The listing builds one solid part. Answer for the finished solid, in the listing's coordinates (mm). A direction names the side the tool comes from. Coordinates: 2 decimals unless noted, no trailing zeros. Order: outer loops, then holes, each group sorted by start corner. A loop starts at its lowest first (then second) coordinate and runs counter-clockwise, first axis right, second up. Notation, with made-up numbers: (-33, 58.5) -> (7, 58.5) arc R29 cw to (7, 89.5) -> close; hole circle Ø2 at (-3.75, -38). An arc over 180 degrees is marked (long way). Write item = value, one per line.
from build123d import *

# Parameters (mm, degrees)
CUT_EXTRUDE_1_DEPTH = 0.75


with BuildPart() as part:
    # 草图1 → 旋转1 (revolve)
    with BuildSketch(Plane.XY):
        Polygon((0, 0), (0, 1.25), (-9.75, 1.25), (-9.75, 0.875), (-10.5, 0.875), (-11.8, 2.35), (-12, 2.35), (-12, 0), align=None)
    revolve(axis=Axis((0, 0, 0), (-1, 0, 0)))

    # 草图2 → 切除-拉伸1 (cut)
    with BuildSketch(Plane.ZY.offset(12)):
        with BuildLine():
            Line((-0.3125, 1.5), (0.3125, 1.5))
            Line((0.3125, 1.5), (0.3125, 0.5625))
            ThreePointArc((0.3125, 0.5625), (0.385723305, 0.385723305), (0.5625, 0.3125))
            Line((0.5625, 0.3125), (1.5, 0.3125))
            Line((1.5, 0.3125), (1.5, -0.3125))
            Line((1.5, -0.3125), (0.5625, -0.3125))
            ThreePointArc((0.5625, -0.3125), (0.385723305, -0.385723305), (0.3125, -0.5625))
            Line((0.3125, -0.5625), (0.3125, -1.5))
            Line((0.3125, -1.5), (-0.3125, -1.5))
            Line((-0.3125, -1.5), (-0.3125, -0.5625))
            ThreePointArc((-0.3125, -0.5625), (-0.385723305, -0.385723305), (-0.5625, -0.3125))
            Line((-0.5625, -0.3125), (-1.5, -0.3125))
            Line((-1.5, -0.3125), (-1.5, 0.3125))
            Line((-1.5, 0.3125), (-0.5625, 0.3125))
            ThreePointArc((-0.5625, 0.3125), (-0.385723305, 0.385723305), (-0.3125, 0.5625))
            Line((-0.3125, 0.5625), (-0.3125, 1.5))
        make_face()
    extrude(amount=-CUT_EXTRUDE_1_DEPTH, mode=Mode.SUBTRACT)


solid = part.part
Q1. Each of these flat-tipped pins is pushed along its axis until it touches: pin 1 Ø2 at (x, y) = (-7, 0.5) entering from +Z; pin 2 Ø0.6 at (x, y) = (-11.5, 1) entering from -Z; pin 3 Ø0.5 at (x, y) = (-11.5, 0) entering from -Z. Where does it stop, or does it pass through?
The answers:
pin_1 = 1.25
pin_2 = -2.15
pin_3 = -2.29
Q2. Section C-C, the plane x = -6 is taken. Give the vertices of the cut face in (y, z).
The answers:
outline = circle Ø2.5 at (0, 0)
Q3. Find the intervals of material crossed by line 1 along Y through (x, z) = (-11.5, 1.25); line 2 along X through (y, z) = (-0.2, -1.05); line 3 along Y through (x, z) = (-8.75, 0), in increasing order.
The answers:
line_1 = -1.57 to -0.31, 0.31 to 1.57
line_2 = -11.25 to -10.67, -9.75 to 0
line_3 = -1.25 to 1.25
Q4. The mould has two halves that part along Z. Classify faces 3 (the face through (0, 0, 0)), 4 (the face through (-11.25, 0, 0)), 5 (the face through (-4.94, -0.27, 1.22)): released by +Z, released by -Z, zero draft, split by the parting line, or undercut.
The answers:
face_3 = zero draft
face_4 = undercut
face_5 = split by the parting line
Q5. A tool of negligible diameter and unlimited length cuts with its end or side. For faces 1 (the face through (-12, 0.5, 0.5)), 2 (the face through (-10.13, 0.808, 0.335)), from which of +Z, -Z, +X, -X, +Y, -Y can it reach the whole face along a straight path? Write none if from no direction.
The answers:
face_1 = +Z, -Z, -X, +Y, -Y
face_2 = none
Q6. Section D-D, the plane x = -10.75 is taken. Give the vertices of the cut face in (y, z), plus the area to 3 significant figures.
The answers:
outline = circle Ø2.32 at (0, 0)
area = 4.22 mm2
Q7. Section A-A, the plane z = 0 is taken. Give the vertices of the cut face in (x, y) (3 decimals), plus the area to 3 significant figures.
The answers:
outline = (-12, -2.35) -> (-11.8, -2.35) -> (-10.5, -0.875) -> (-9.75, -0.875) -> (-9.75, -1.25) -> (0, -1.25) -> (0, 1.25) -> (-9.75, 1.25) -> (-9.75, 0.875) -> (-10.5, 0.875) -> (-11.8, 2.35) -> (-12, 2.35) -> (-12, 1.5) -> (-11.25, 1.5) -> (-11.25, -1.5) -> (-12, -1.5) -> close
area = 28.6 mm2
